```python
from build123d import *

# Parameters (mm, degrees)
F1_DEPTH = 19.05
F2_R     = 2.15265
F2_R_2   = 1.7272
F3_DEPTH = 9.525


with BuildPart() as f1:
    # F0 (on Top) → F1 (new body)
    with BuildSketch(Plane.XY):
        Polygon((0, 0), (0, 6.35), (9.525, 6.35), (9.525, 0), (23.8125, 0), (23.8125, 3.175), (14.2875, 3.175), (14.2875, 9.525), (-4.7625, 9.525), (-4.7625, 3.175), (-14.2875, 3.175), (-14.2875, 0), align=None)
    extrude(amount=F1_DEPTH)

    # F2 (on face) → F3 (cut, through all)
    with BuildSketch(Plane.XZ):
        with Locations((4.7625, 4.7625)):
            Circle(F2_R)
        with Locations((4.7625, 14.2875)):
            Circle(F2_R)
        with Locations((-9.525, 9.525)):
            Circle(F2_R_2)
        with Locations((19.05, 9.525)):
            Circle(F2_R_2)
    extrude(amount=-F3_DEPTH, mode=Mode.SUBTRACT)


solid = f1.part
```
Can you work these out from the model? Positions are in its coordinate system, mm. A direction names the side the tool comes from. Coordinates: 2 decimals unless noted, no trailing zeros. Order: outer loops, then holes, each group sorted by start corner. A loop starts at its lowest first (then second) coordinate and runs counter-clockwise, first axis right, second up. Notation, with made-up numbers: (60.5, 67.5) - (108.5, 67.5) arc R4 ccw to (108.5, 71.5) - close; hole circle Ø3 at (21.5, -14.75). An arc over 180 degrees is marked (long way). Answer in a Markdown table with one row per item.
1. If I drill on line 1 along X through (y, z) = (7.5, 15.75); line 2 along Z through (x, y) = (19.05, 1.7); line 3 along X through (y, z) = (2.25, 10.25) (1 decimal), over which ranges is the centre line in solid material (lowest first)?
Reply:
| item | result |
|---|---|
| line 1 | x = -4.76 to 3.18, 6.34 to 14.29 |
| line 2 | z = 0 to 7.8, 11.25 to 19.05 |
| line 3 | x = -14.3 to -11.1, -8 to 0, 9.5 to 17.5, 20.6 to 23.8 |
2. For faces 1 (the flat face through (-9, 3.175, 12)), 2 (the flat face through (21, 3.175, 9)), 3 (the flat face through (9.525, 3, 9)), which set-ups out of +Z, -Z, +X, -X, +Y, -Y let a thin tool reach every point of the face, with its end or its side?
Reply:
| item | result |
|---|---|
| face 1 | +Z, -Z, -X, +Y |
| face 2 | +Z, -Z, +X, +Y |
| face 3 | +Z, -Z, -Y |
3. If we mould it in two halves opening along Z, with no side actions, what happens to faces 4 (the flat face through (4, 7, 0)), 5 (the flat face through (-4.762, 6, 9)), 6 (the cylindrical face through (-7.878, 1.565, 10.044))? For each: pulls with the +Z half, pulls with the -Z half, needs draft (parallel to the pull), parting line crosses it, or undercut.
Reply:
| item | result |
|---|---|
| face 4 | pulls with the -Z half |
| face 5 | needs draft |
| face 6 | undercut |
4. Suppose I cut it at C-C (x = 19.05). Please give me the cut outline in (y, z) (3 decimals), and give its area (3 significant figures).
Reply:
| item | result |
|---|---|
| outline | (0, 0) - (3.175, 0) - (3.175, 7.798) - (0, 7.798) - close; (0, 11.252) - (3.175, 11.252) - (3.175, 19.05) - (0, 19.05) - close |
| area | 49.5 mm^2 |
5. Suppose I cut it at B-B (y = 0.5). Give the number of separate pieces and of enclosed holes in the cut face, and give its area (3 significant figures).
Reply:
| item | result |
|---|---|
| separate pieces | 2 |
| enclosed holes | 2 |
| area | 526 mm^2 |
6. For pin 1 (5 mm diameter, centred on x = 4.76, z = 14.29, fed in from -Y); pin 2 (4.5 mm diameter, centred on x = -9.525, z = 9.525, fed in from +Y) (3 decimals); pin 3 (3 mm diameter, centred on y = 5, z = 8.5, fed in from +X), each with a flat end and sliding along its axis, tell me the tip position at first contact or that it passes through.
Reply:
| item | result |
|---|---|
| pin 1 | stops at y = 6.35 |
| pin 2 | stops at y = 3.175 |
| pin 3 | stops at x = 14.29 |
